Check sheet for the modelled part. Datum: model origin and axes. Units: mm. A direction names the side the tool comes from. Give positions to 0.01 mm unless a question says otherwise; leave off trailing zeros. Write each loop counter-clockwise with the first axis right and the second up, starting at its lowest first coordinate (ties: lowest second). Pieces come first, ordered by that corner, then holes. Notation, with made-up numbers: M 62.5,69 L 111.5,69 A18 cw 111.5,92 Z; hole C 19,-27.75 d2. An arc over 180 degrees is marked long. One line per item, written item: value. Start each with the question number.
from build123d import *

# Parameters (mm, degrees)
F0_W     = 0.5
F0_H     = 29.5
F0_W_2   = 29
F0_H_2   = 0.5
F1_DEPTH = 600


with BuildPart() as f1:
    # F0 (on Top) → F1 (new body)
    with BuildSketch(Plane.XY):
        with Locations((1.0650282837, -3.191780895)):
            Rectangle(F0_W, F0_H)
        with Locations((15.8150282837, -18.191780895)):
            Rectangle(F0_W_2, F0_H_2)
        with Locations((30.5650282837, -3.191780895)):
            Rectangle(F0_W, F0_H)
        with Locations((30.5650282837, -18.191780895)):
            Rectangle(F0_W, F0_H_2)
        with Locations((1.0650282837, -18.191780895)):
            Rectangle(F0_W, F0_H_2)
    extrude(amount=F1_DEPTH)


solid = f1.part
1) Tool access check on faces 4 (the flat face through (30.315, -3, 296)), 5 (the flat face through (16, -18.442, 296)). Record the directions out of +Z, -Z, +X, -X, +Y, -Y that give a thin tool (end or side, any length) a straight path to the whole face; none if there is none.
2) Draft check along X on faces 1 (the flat face through (1, -3, 600)), 2 (the flat face through (30.815, -4, 296)), 3 (the flat face through (16, -17.942, 296)). Enter one of: released by +X, released by -X, zero draft, split by the parting line, or undercut.
3) Cross-section at A-A (y = -8). Record the boundary of the cut face in (x, z), plus the area to 3 significant figures.
4) Cross-section at C-C (x = 9.5). Record the boundary of the cut face in (y, z).
5) Cross-section at B-B (z = 302). Record the boundary of the cut face in (x, y).
6) Gauge pin test, flat end, axial feed: pin 1 (14.5 mm diameter, centred on x = 15.5, z = 286.5, fed in from +Y). Record the tip position at first contact, or that the pin passes through.
7) Material ranges on L1, parallel to X at y = 0.25, z = 300; L2, parallel to Y at x = 21, z = 369.5, recorded low to high. Write a range as from..to.
Data:
1. face 4: +Z, -Z, +Y
1. face 5: +Z, -Z, +X, -X, -Y
2. face 1: zero draft
2. face 2: released by +X
2. face 3: undercut
3. outline: M 0.82,0 L 1.32,0 L 1.32,600 L 0.82,600 Z; M 30.32,0 L 30.82,0 L 30.82,600 L 30.32,600 Z
3. area: 600 mm2
4. outline: M -18.44,0 L -17.94,0 L -17.94,600 L -18.44,600 Z
5. outline: M 0.82,-18.44 L 30.82,-18.44 L 30.82,11.56 L 30.32,11.56 L 30.32,-17.94 L 1.32,-17.94 L 1.32,11.56 L 0.82,11.56 Z
6. pin 1: stops at y = -17.94
7. L1: x = 0.82..1.32, 30.32..30.82
7. L2: y = -18.44..-17.94
